from build123d import *

# Parameters (mm, degrees)
CYLINDER_R        = 10.2
CYLINDER_DEPTH    = 18
CYLINDER001_R     = 11.7
CYLINDER001_DEPTH = 3


with BuildPart() as cilindro_interior:
    # Cylinder → Cylinder (new body)
    with BuildSketch(Plane.XY.offset(-8)):
        Circle(CYLINDER_R)
    extrude(amount=CYLINDER_DEPTH)


with BuildPart() as obj1:
    # Cylinder001 → Cylinder001 (new body)
    with BuildSketch(Plane.XY):
        Circle(CYLINDER001_R)
    extrude(amount=CYLINDER001_DEPTH)

    # Cut: cut cilindro-interior
    add(cilindro_interior.part, mode=Mode.SUBTRACT)


solid = obj1.part
For this review, take the finished solid that the model builds, in its own axes (mm). Coordinates: 2 decimals unless noted, no trailing zeros. Order: outer loops, then holes, each group sorted by start corner. A loop starts at its lowest first (then second) coordinate and runs counter-clockwise, first axis right, second up. Notation, with made-up numbers: (-2.75, -23) - (31.25, -23) arc R24 cw to (31.25, 8) - close; hole circle Ø2 at (27.25, 84.25). An arc over 180 degrees is marked (long way). Use one line per item in the form item = value.
Q1. Consider section C-C (z = 2.25). Give the boundary of the cut face in (x, y).
Checked values:
outline = circle Ø23.4 at (0, 0); hole circle Ø20.4 at (0, 0)
Q2. For probe 1 along Y at (x, z) = (0, 2.15); probe 2 along X at (y, z) = (-2.5, 2.65); probe 3 along X at (y, z) = (-9, 0.9), list the stretches that pass through material, from the lowest coordinate up. Write a range as from..to.
Checked values:
probe_1 = -11.7..-10.2, 10.2..11.7
probe_2 = -11.43..-9.89, 9.89..11.43
probe_3 = -7.48..-4.8, 4.8..7.48
Q3. Draft analysis for pull direction Y (two halves, no side actions). For faces 1 (the cylindrical face through (4.707, -9.049, 1.479)), 2 (the cylindrical face through (-2.54, -11.42, 1.48)), 3 (the flat face through (-4, 10, 3)), state which applies: +Y half, -Y half, draft (parallel to the pull), parting line (faces both ways), or undercut.
Checked values:
face_1 = undercut
face_2 = parting line
face_3 = draft
Q4. Consider section A-A (x = 0). Give the boundary of the cut face in (y, z).
Checked values:
outline = (-11.7, 0) - (-10.2, 0) - (-10.2, 3) - (-11.7, 3) - close; (10.2, 0) - (11.7, 0) - (11.7, 3) - (10.2, 3) - close
Q5. For P1, Ø10, axis at x = -5.5, y = -3.5, coming from the -Z side; P2, Ø6, axis at x = 2, y = -4.5, coming from the +Z side; P3, Ø1, axis at y = 8, z = 2.5, coming from the -X side; P4, Ø1.5, axis at y = -1, z = 2.5, coming from the +X side, all flat-tipped, find the tip position at first contact; note any pin that passes through.
Checked values:
P1 = 0
P2 = through
P3 = -8.98
P4 = 11.7
